Here's the drawing with two shaded views (mm, measured from the low corner). I have some questions. A direction names the side the tool comes from. Give positions to 0.01 mm unless a question says otherwise; leave off trailing zeros. Loops run counter-clockwise (first coordinate to the right, second up) from the corner with the lowest first, then second, coordinate; pieces in that order, holes last. Notation, with made-up numbers: M 17,71 L 44,71 A28 cw 44,104 Z; hole C -14,85.25 d3. An arc over 180 degrees is marked long. Write item = value, one per line. Start each with the question number.
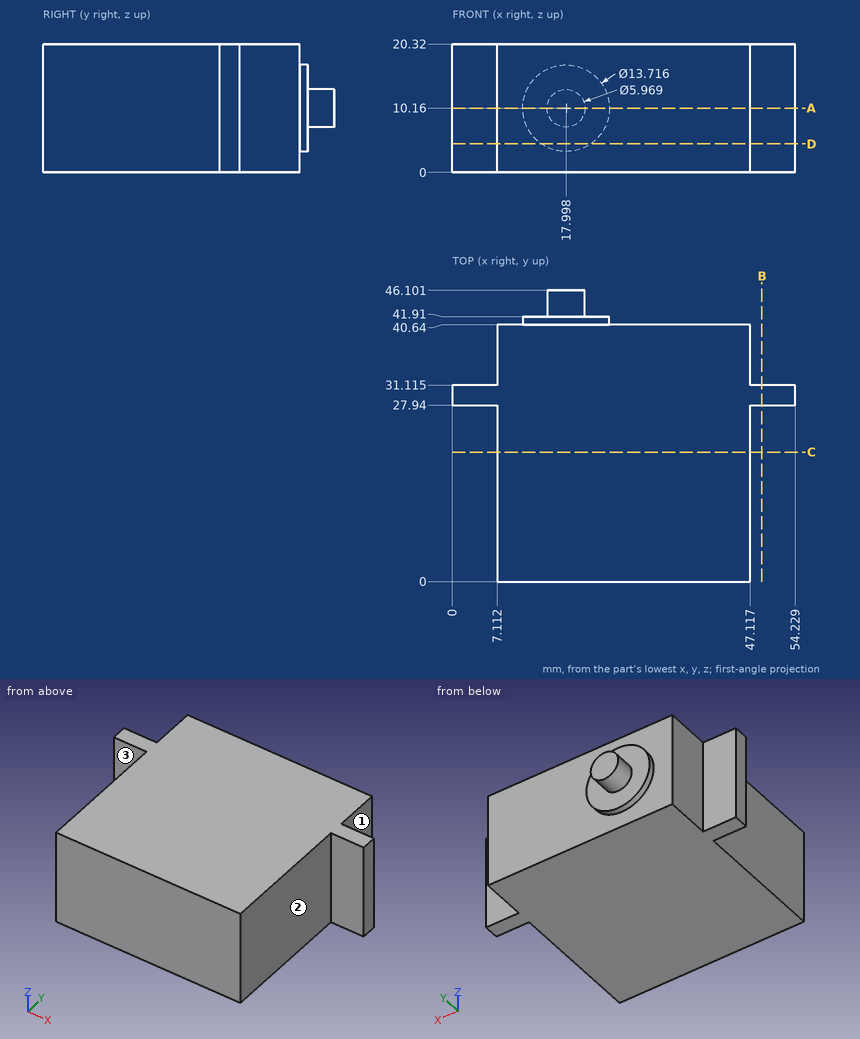
Q1. If we section it at C-C, the plane y = 20.5: List the corners of the cut face in (x, z) for me.
Q2. Will these pins go through, and if not, where does the flat tip stop? pin 1 (2 mm diameter, centred on x = 33, y = 35, fed in from -Z); pin 2 (2 mm diameter, centred on x = 49.5, z = 7.5, fed in from -Y); pin 3 (5.5 mm diameter, centred on x = 50.5, z = 6, fed in from +Y) (3 decimals); pin 4 (10.5 mm diameter, centred on y = 36.5, z = 14, fed in from -X).
Q3. If we section it at B-B, the plane x = 49: List the corners of the cut face in (y, z) for me (1 decimal).
Q4. If I drill on line 1 along Y through (x, z) = (6, 12.5) (1 decimal); line 2 along X through (y, z) = (40.5, 3.25); line 3 along Y through (x, z) = (28.5, 4), over which ranges is the centre line in solid material (lowest first)?
Q5. If we section it at D-D, the plane z = 4.5: List the corners of the cut face in (x, y) for me (1 decimal).
Q6. If we section it at A-A, the plane z = 10.16: List the corners of the cut face in (x, y) for me (1 decimal).
Q7. On a 3-axis mill with a long thin cutter (end or side, diameter ignored), from which of +Z, -Z, +X, -X, +Y, -Y can I reach the whole of each face in a straight line? I mean the marked faces 1, 2 and 3. Say none if no direction works.
Resolved:
q1.outline = M 7.11,0 L 47.12,0 L 47.12,20.32 L 7.11,20.32 Z
q2.pin_1 = 0
q2.pin_2 = 27.94
q2.pin_3 = 31.115
q2.pin_4 = 7.11
q3.outline = M 27.9,0 L 31.1,0 L 31.1,20.3 L 27.9,20.3 Z
q4.line_1 = 27.9 to 31.1
q4.line_2 = 7.11 to 47.12
q4.line_3 = 0 to 40.64
q5.outline = M 0,27.9 L 7.1,27.9 L 7.1,0 L 47.1,0 L 47.1,27.9 L 54.2,27.9 L 54.2,31.1 L 47.1,31.1 L 47.1,40.6 L 21.9,40.6 L 21.9,41.9 L 14.1,41.9 L 14.1,40.6 L 7.1,40.6 L 7.1,31.1 L 0,31.1 Z
q6.outline = M 0,27.9 L 7.1,27.9 L 7.1,0 L 47.1,0 L 47.1,27.9 L 54.2,27.9 L 54.2,31.1 L 47.1,31.1 L 47.1,40.6 L 24.9,40.6 L 24.9,41.9 L 21,41.9 L 21,46.1 L 15,46.1 L 15,41.9 L 11.1,41.9 L 11.1,40.6 L 7.1,40.6 L 7.1,31.1 L 0,31.1 Z
q7.face_1 = +Z, -Z, +X, +Y
q7.face_2 = +Z, -Z, +X, -Y
q7.face_3 = +Z, -Z, -X, -Y
